Autodesk Inventor part; units mm, degrees
ref_plane "YZ Plane" through (0, 0, 0) normal (1, 0, 0) x (0, 1, 0)
ref_plane "XZ Plane" through (0, 0, 0) normal (0, 1, 0) x (-1, 0, 0)
ref_plane "XY Plane" through (0, 0, 0) normal (0, 0, 1) x (1, 0, 0)
sketch "Sketch1" plane through (0, 0, 0) normal (0, 1, 0) x (-1, 0, 0)
  line L0 (13.7338, 24.3615) -> (-17.2662, 24.3615)
  line L1 (-17.2662, 24.3615) -> (-17.2662, -45.6385)
  line L2 (-17.2662, -45.6385) -> (13.7338, -45.6385)
  line L3 (13.7338, -45.6385) -> (13.7338, 24.3615)
  point P0 (0, 0)
  dimension "d0" = 31
  dimension "d1" = 70
extrude "Extrusion1" add sketch "Sketch1" along normal blind 54.75
sketch "Sketch2" plane through (17.2662, 0, 24.3615) normal (1, 0, 0) x (0, 0, -1)
  circle A0 centre (35, 35.9173) radius 27.375
  line L0 (0, 54.75) -> (70, 54.75) construction
  point P0 (24.3615, 0)
  point P1 (35, 54.75)
  dimension "d4" = 54.75
hole "Hole1" at (17.2662, 35.9173, -10.6385) direction (-1, 0, 0) diameter 54.75 end through all
sketch "Sketch3" plane through (0, 0, 0) normal (0, -1, 0) x (1, 0, 0)
  point P0 (0, 0)
sketch "Sketch4" plane through (0, 54.75, 0) normal (0, 1, 0) x (1, 0, 0)
  line L0 (-13.7338, -9.229) -> (17.2662, -9.229) construction
  line L1 (17.2662, -9.229) -> (-13.7338, -9.229) construction
  circle A0 centre (1.7662, -9.229) radius 4 construction
  point P0 (0, 0)
  dimension "d12" = 8
sketch "Sketch5" plane through (0, 54.75, 0) normal (0, 1, 0) x (1, 0, 0)
  line L0 (17.2662, 30.506) -> (-13.7338, 30.506) construction
  line L1 (-13.7338, 30.506) -> (17.2662, 30.506) construction
  circle A0 centre (1.7662, 30.506) radius 4 construction
  point P0 (0, 0)
  dimension "d13" = 8
hole "Hole2" at (1.7662, 54.75, 9.229) direction (0, -1, 0) diameter 8 depth 8 tip angle 118
hole "Hole3" at (1.7662, 54.75, -30.506) direction (0, -1, 0) diameter 8 depth 8 tip angle 118
sketch "Sketch6" plane through (0, 54.75, 0) normal (0, 1, 0) x (1, 0, 0)
  point P0 (0, 0)
properties part number "Noke_base"
Source: CAD feature listing. Evaluate the final solid. Frame: model axes, mm. A direction names the side the tool comes from. Round coordinates to 2 decimals unless told otherwise and drop trailing zeros. Write each loop counter-clockwise with the first axis right and the second up, starting at its lowest first coordinate (ties: lowest second). Pieces come first, ordered by that corner, then holes. Notation, with made-up numbers: M 79.25,85.25 L 90.25,85.25 A13 ccw 90.25,108.25 Z; hole C 10,43 d5. An arc over 180 degrees is marked long. Use CSV: the item, a comma, the result in double quotes. Start each with the question number.
Q1. Line query: line 1 (Z direction, x = -5, y = 52.5); line 2 (Z direction, x = -4.5, y = 23.5); line 3 (Y direction, x = -6.5, z = -11.5). Output: solid intervals per line, ascending. Write a range as from..to.
Q2. Cut plane D-D on z = 8. Output: boundary loops of the cut face in (x, y), plus the area to 3 significant figures.
Q3. First-contact query: P1, Ø8, axis at x = 0, z = -32.5, coming from the +Y side. Flat tip, straight axial feed; report the tip coordinate or a pass-through.
Q4. Access query for faces 1 (the face through (2, 54.75, 17)), 2 (the face through (1.678, 52.601, -34.505)). Directions: +Z, -Z, +X, -X, +Y, -Y. A direction counts if a zero-diameter tool reaches every point of the face in a straight line with its end or side. Return the directions, or none.
Q5. Cut plane C-C on y = 32. Output: boundary loops of the cut face in (x, z).
Q6. Pull-direction query (Z, two-part tool) for faces 3 (the face through (2, 0, -10)), 4 (the face through (2, 27, -45.638)), 5 (the face through (1.85, 52.6, 13.23)); classes: +Z half, -Z half, draft (parallel to the pull), parting line (faces both ways), or undercut.
Q7. Cut plane A-A on y = 44. Output: boundary loops of the cut face in (x, z).
Results found:
1,line 1,"-45.64..-32.42, 11.14..24.36"
1,line 2,"-45.64..-35.04, 13.76..24.36"
1,line 3,"0..8.56"
2,outline,"M -13.73,0 L 17.27,0 L 17.27,15.87 L -13.73,15.87 Z"
2,area,"492 mm^2"
3,P1,"y = 54.75"
4,face 1,"+Z, -Z, +X, -X, +Y"
4,face 2,"+Y"
5,outline,"M -13.73,-45.64 L 17.27,-45.64 L 17.27,-37.73 L -13.73,-37.73 Z; M -13.73,16.45 L 17.27,16.45 L 17.27,24.36 L -13.73,24.36 Z"
6,face 3,"draft"
6,face 4,"-Z half"
6,face 5,"undercut"
7,outline,"M -13.73,-45.64 L 17.27,-45.64 L 17.27,-36.79 L -13.73,-36.79 Z; M -13.73,15.52 L 17.27,15.52 L 17.27,24.36 L -13.73,24.36 Z"
